Design review of the part built by this model. Coordinates are the model's own, in mm. Round coordinates to 2 decimals unless told otherwise and drop trailing zeros. Loops run counter-clockwise (first coordinate to the right, second up) from the corner with the lowest first, then second, coordinate; pieces in that order, holes last. Notation, with made-up numbers: (23, -5.75) -> (29, -5.75) arc R24 ccw to (29, 25.25) -> close; hole circle Ø11 at (13.5, 81.5). An arc over 180 degrees is marked (long way). Write each question's results on one line, items separated by ' | '. Start each with the question number.
Autodesk Inventor part; units mm, degrees
ref_plane "YZ Plane" through (0, 0, 0) normal (1, 0, 0) x (0, 1, 0)
ref_plane "XZ Plane" through (0, 0, 0) normal (0, 1, 0) x (-1, 0, 0)
ref_plane "XY Plane" through (0, 0, 0) normal (0, 0, 1) x (1, 0, 0)
sketch "Sketch2" plane through (0, 0, 0) normal (0, 1, 0) x (-1, 0, 0)
  line L0 (0, -28.76) -> (0, 88.56) construction
  circle A0 centre (0, 64.8) radius 4
  arc A1 (4, 59.0554) -> (-4, 59.0554) centre (0, 64.8) ccw
  line L1 (-4, 59.0554) -> (-11.8883, 1.6332)
  line L2 (11.8883, 1.6332) -> (4, 59.0554)
  circle A2 centre (0, 0) radius 9
  arc A3 (-11.8883, 1.6332) -> (11.8883, 1.6332) centre (0, 0) ccw
  dimension "d7" = 3
  dimension "d8" = 8
  dimension "d22" = 64.8
  dimension "d25" = 3
  dimension "d26" = 18
  dimension "d27" = 8
extrude "Extrusion1" add sketch "Sketch2" along normal blind 4
properties part number "P012" material "Iron, Gray"
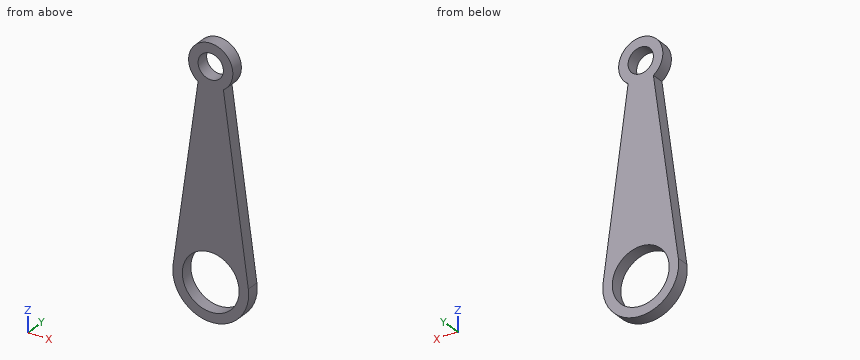
1) Take a section at B-B (z = 64.8). Write out the cut boundary in (x, y), plus the area to 3 significant figures.
2) To check wall thickness, follow line 1 (X direction, y = 2.7, z = -8); line 2 (X direction, y = 1.55, z = 36.5); line 3 (X direction, y = 1.2, z = 5). State the ranges of each line that lie inside material, in increasing order. Write a range as from..to.
3) Insertion check: pin 1 (10.5 mm diameter, centred on x = 0, z = 64.8, fed in from +Y); pin 2 (1 mm diameter, centred on y = 2, z = 53.5, fed in from +X). Each pin has a flat end and moves straight along its axis. Give the tip position at first contact, or say it passes through.
4) Take a section at D-D (x = 7.75). Write out the cut boundary in (y, z).
5) Take a section at A-A (x = 0). Write out the cut boundary in (y, z).
6) Take a section at C-C (y = 0.9). Write out the cut boundary in (x, z).
Geometry check:
1) outline: (-7, 0) -> (-4, 0) -> (-4, 4) -> (-7, 4) -> close; (4, 0) -> (7, 0) -> (7, 4) -> (4, 4) -> close | area: 24.0 mm^2
2) line 1: x = -8.94..-4.12, 4.12..8.94 | line 2: x = -7.1..7.1 | line 3: x = -11.43..-7.48, 7.48..11.43
3) pin 1: stops at y = 4 | pin 2: stops at x = 4.83
4) outline: (0, -9.16) -> (4, -9.16) -> (4, -4.58) -> (0, -4.58) -> close; (0, 4.58) -> (4, 4.58) -> (4, 31.76) -> (0, 31.76) -> close
5) outline: (0, -12) -> (4, -12) -> (4, -9) -> (0, -9) -> close; (0, 9) -> (4, 9) -> (4, 60.8) -> (0, 60.8) -> close; (0, 68.8) -> (4, 68.8) -> (4, 71.8) -> (0, 71.8) -> close
6) outline: (-11.89, 1.63) arc R12 ccw (long way) to (11.89, 1.63) -> (4, 59.06) arc R7 ccw (long way) to (-4, 59.06) -> close; hole circle Ø18 at (0, 0); hole circle Ø8 at (0, 64.8)
